Part print with two shaded views. Sizes in mm from the minimum x, y, z corner. Round coordinates to 2 decimals unless told otherwise and drop trailing zeros. Order: outer loops, then holes, each group sorted by start corner. A loop starts at its lowest first (then second) coordinate and runs counter-clockwise, first axis right, second up. Notation, with made-up numbers: (-10, 27) -> (4, 27) arc R22 ccw to (4, 48) -> close; hole circle Ø3 at (83.5, 57.5). An arc over 180 degrees is marked (long way). Put each result on its own line as item: value. Start each with the question number.
Q1. Flat gauge pin, fed straight in: P1, Ø3, axis at y = 4, z = 1.5, coming from the +X side. Where does the tip first touch, or does it go through?
Q2. Cut at B-B, the plane x = 8.5. List the corners of the cut face in (y, z).
Q3. Cut at A-A, the plane x = 4.75. List the corners of the cut face in (y, z), and give its area (3 significant figures).
Q4. Probe L1, parallel to Z at x = 6, y = 1.8; L2, parallel to Z at x = 7.5, y = 4; L3, parallel to X at y = 4.5, z = 1.95 (1 decimal). List the from-to ranges inside material, lowest first.
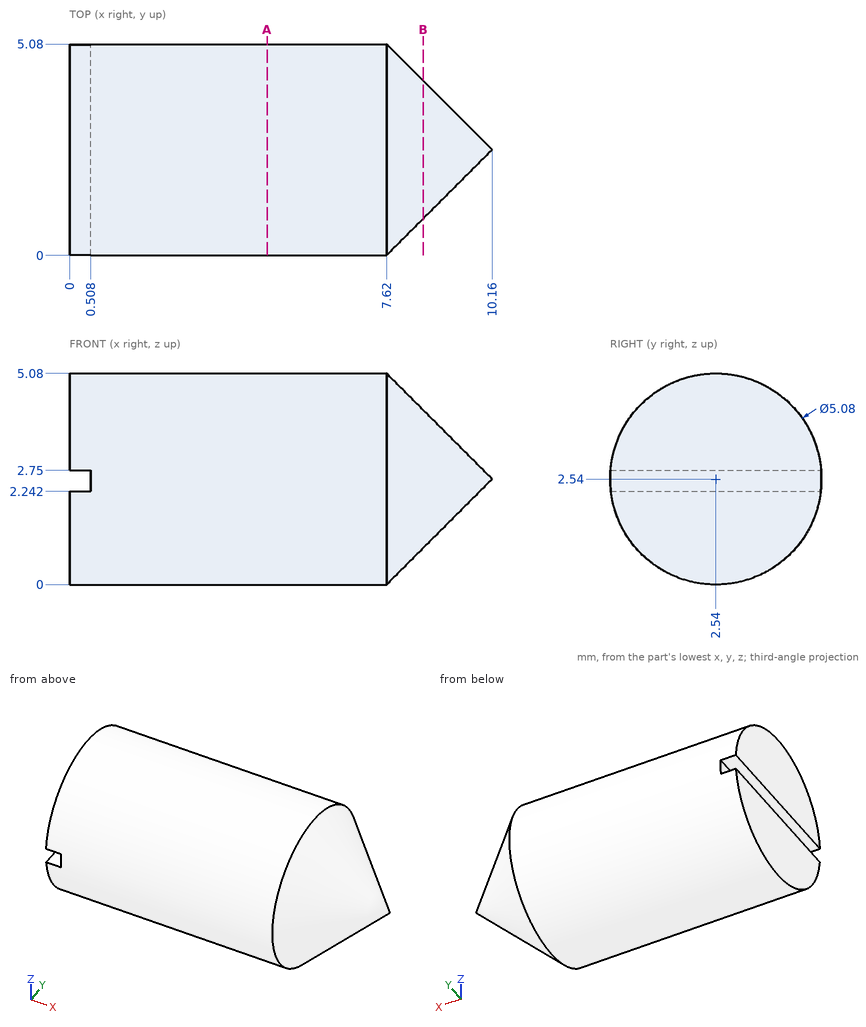
Ans:
1. P1: stops at x = 9.87
2. outline: circle Ø3.32 at (2.54, 2.54)
3. outline: circle Ø5.08 at (2.54, 2.54)
3. area: 20.3 mm^2
4. L1: z = 0.11 to 4.97
4. L2: z = 0.46 to 4.62
4. L3: x = 0 to 8.1
